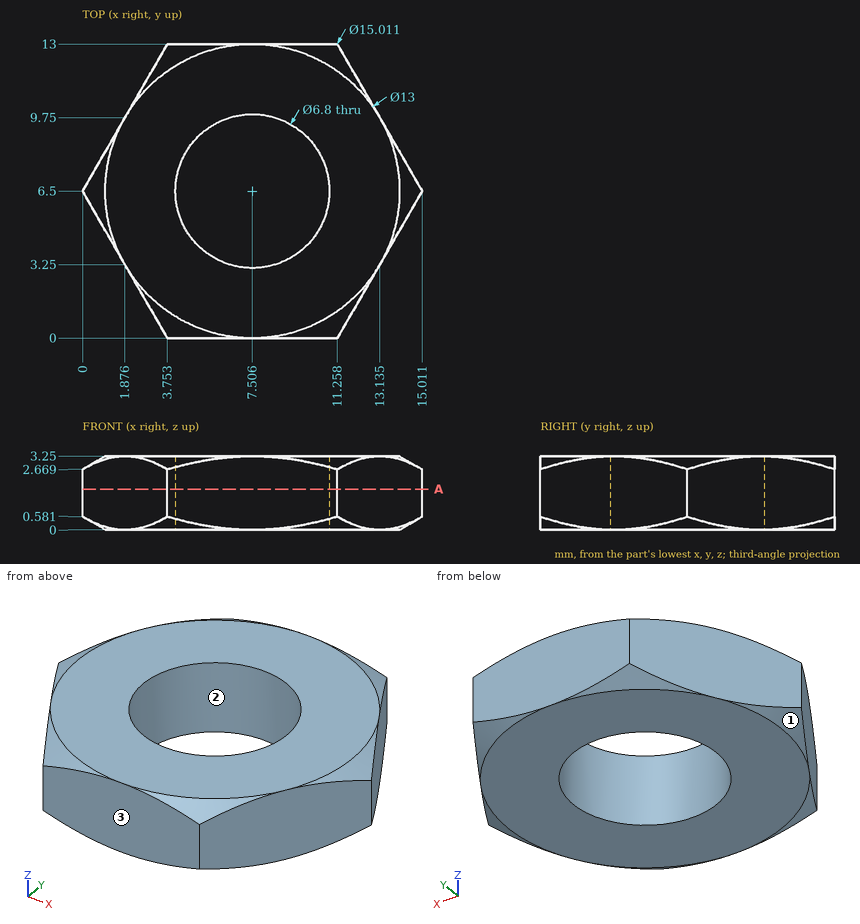
The figure shows three views and two pictorial views of one solid part (mm, origin at its lowest corner). Answer the questions. Round coordinates to 2 decimals unless told otherwise and drop trailing zeros. Write each loop counter-clockwise with the first axis right and the second up, starting at its lowest first coordinate (ties: lowest second). Pieces come first, ordered by that corner, then holes. Notation, with made-up numbers: M -30,81 L 12,81 A27 cw 12,109 Z; hole C -40,71 d1. An arc over 180 degrees is marked long. Use a Markdown table: item, result.
1) The part is cut by section A-A on z = 1.8. Give the vertices of the cut face in (x, y) (1 decimal).
Taken from the geometry:
| item | result |
|---|---|
| outline | M 0,6.5 L 3.8,0 L 11.3,0 L 15,6.5 L 11.3,13 L 3.8,13 Z; hole C 7.5,6.5 d6.8 |
2) Determine the mould class of the marked faces 1, 2 and 3 for opening direction Y: pulls with the +Y half, pulls with the -Y half, needs draft (parallel to the pull), parting line crosses it, or undercut.
Taken from the geometry:
| item | result |
|---|---|
| face 1 | parting line crosses it |
| face 2 | undercut |
| face 3 | pulls with the -Y half |
3) Flat-ended cylindrical pins translate along their axes: pin 1 (1.5 mm diameter, centred on y = 6, z = 0.5, fed in from -X); pin 2 (1.5 mm diameter, centred on y = 10, z = 2, fed in from +X). Find the tip coordinate at first contact, or state that the pin passes through.
Taken from the geometry:
| item | result |
|---|---|
| pin 1 | stops at x = 0 |
| pin 2 | stops at x = 13.42 |
4) Consider line 1 (Y direction, x = 6.25, z = 2.35); line 2 (Y direction, x = 8.25, z = 1.95); line 3 (X direction, y = 5.5, z = 2.8) (1 decimal). Determine where each line is inside the solid, lowest interval first. Write a range as [from, to].
Taken from the geometry:
| item | result |
|---|---|
| line 1 | y = [0, 3.34], [9.66, 13] |
| line 2 | y = [0, 3.18], [9.82, 13] |
| line 3 | x = [0.6, 4.3], [10.8, 14.4] |
